from build123d import *

# Parameters (mm, degrees)
F0_W     = 152.4
F0_H     = 66.074036
F0_R     = 12.7
F1_DEPTH = 20.32
F2_DEPTH = 52.07


with BuildPart() as f1:
    # F0 (on Top) → F1 (new body)
    with BuildSketch(Plane.XY):
        with Locations((-31.75, 0)):
            Rectangle(F0_W, F0_H)
        Polygon((-6.35, -21.997045), (6.35, 0), (19.05, -21.997045), align=None, mode=Mode.SUBTRACT)
        with Locations((-82.55, 0)):
            Circle(F0_R, mode=Mode.SUBTRACT)
        Polygon((-22.225, 9.525), (-22.225, 0), (-22.225, -9.525), (-41.275, -9.525), (-41.275, 0), (-41.275, 9.525), align=None, mode=Mode.SUBTRACT)
    extrude(amount=-F1_DEPTH)

    # F0 (on Top) → F2 (join)
    with BuildSketch(Plane.XY):
        Polygon((-22.225, -9.525), (-22.225, 0), (-31.75, 0), (-41.275, 0), (-41.275, -9.525), align=None)
        Polygon((-31.75, 0), (-22.225, 0), (-22.225, 9.525), (-41.275, 9.525), (-41.275, 0), align=None)
        with Locations((-82.55, 0)):
            Circle(F0_R)
    extrude(amount=-F2_DEPTH)


solid = f1.part
CAD build for the part. Positions are in the model's coordinates, mm. A direction names the side the tool comes from. Give positions to 0.01 mm unless a question says otherwise; leave off trailing zeros. Write each loop counter-clockwise with the first axis right and the second up, starting at its lowest first coordinate (ties: lowest second). Pieces come first, ordered by that corner, then holes. Notation, with made-up numbers: (61.5, 0) -> (93.5, 0) arc R30 cw to (93.5, 38) -> close; hole circle Ø8 at (8, 13.5). An arc over 180 degrees is marked (long way). Return JSON: item names as keys, results as strings.
Item 1: Tool access for faces 5 (the flat face through (-22.225, 0, -36)), 6 (the flat face through (12.61, -10.84, -10.02)), 7 (the flat face through (-41.275, 0, -36)), 8 (the flat face through (-32, -9.525, -36)): list every direction of +Z, -Z, +X, -X, +Y, -Y with a clear straight run to the whole face (end or side of a thin tool).
Answer below:
{"face 5": "-Z, +X, +Y, -Y", "face 6": "+Z, -Z", "face 7": "-Z, +Y, -Y", "face 8": "-Z, +X, -Y"}
Item 2: Band-saw the part on C-C (y = -1.5). List the corners of the cut face in (x, z) (3 decimals).
Answer below:
{"outline": "(-107.95, -20.32) -> (-95.161, -20.32) -> (-95.161, -52.07) -> (-69.939, -52.07) -> (-69.939, -20.32) -> (-41.275, -20.32) -> (-41.275, -52.07) -> (-22.225, -52.07) -> (-22.225, -20.32) -> (5.484, -20.32) -> (5.484, 0) -> (-107.95, 0) -> close; (7.216, -20.32) -> (44.45, -20.32) -> (44.45, 0) -> (7.216, 0) -> close"}
Item 3: Band-saw the part on A-A (z = -37.5). List the corners of the cut face in (x, y) (3 decimals), then the cut area to 3 significant figures.
Answer below:
{"outline": "circle Ø25.4 at (-82.55, 0); (-41.275, -9.525) -> (-22.225, -9.525) -> (-22.225, 9.525) -> (-41.275, 9.525) -> close", "area": "870 mm2"}
Item 4: Band-saw the part on D-D (x = -82.55). List the corners of the cut face in (y, z), then the cut area to 3 significant figures.
Answer below:
{"outline": "(-33.04, -20.32) -> (-12.7, -20.32) -> (-12.7, -52.07) -> (12.7, -52.07) -> (12.7, -20.32) -> (33.04, -20.32) -> (33.04, 0) -> (-33.04, 0) -> close", "area": "2,150 mm2"}
Item 5: Band-saw the part on B-B (x = -3). List the corners of the cut face in (y, z).
Answer below:
{"outline": "(-33.04, -20.32) -> (-22, -20.32) -> (-22, 0) -> (-33.04, 0) -> close; (-16.19, -20.32) -> (33.04, -20.32) -> (33.04, 0) -> (-16.19, 0) -> close"}
Item 6: Two-plate mould, pull along Y, no slides. Class faces 1 (the flat face through (-33, 0, 0)), 2 (the flat face through (-32, 9.525, -36)), 3 (the flat face through (0, -11, -10)), 4 (the flat face through (7, -21.997, -10)): +Y half, -Y half, draft (parallel to the pull), parting line (faces both ways), or undercut.
Answer below:
{"face 1": "draft", "face 2": "+Y half", "face 3": "undercut", "face 4": "undercut"}
Item 7: Drop flat-ended pins along their axis: pin 1 (6 mm diameter, centred on y = 8, z = -46.5, fed in from -X); pin 2 (5.5 mm diameter, centred on x = -30.5, z = -37, fed in from -Y) (3 decimals); pin 3 (12 mm diameter, centred on x = -88, y = 14.5, fed in from +Z); pin 4 (9.5 mm diameter, centred on y = -3, z = -35, fed in from -X). Give the stop position or say it passes through.
Answer below:
{"pin 1": "stops at x = -94.22", "pin 2": "stops at y = -9.525", "pin 3": "stops at z = 0", "pin 4": "stops at x = -95.25"}
Item 8: Drill centre lines: probe 1 along Z at (x, y) = (-99, 4); probe 2 along X at (y, z) = (-4, -19); probe 3 along X at (y, z) = (-14.5, -5.5). Where is each one in solid material? Low to high.
Answer below:
{"probe 1": "z = -20.32 to 0", "probe 2": "x = -107.95 to 4.04, 8.66 to 44.45", "probe 3": "x = -107.95 to -2.02, 14.72 to 44.45"}
